Work out the finished part from the listing and answer in its coordinate system (mm). Face numbers are marked on the shaded views. A direction names the side the tool comes from. Round coordinates to 2 decimals unless told otherwise and drop trailing zeros. Write each loop counter-clockwise with the first axis right and the second up, starting at its lowest first coordinate (ties: lowest second). Pieces come first, ordered by that corner, then holes.
Autodesk Inventor part; units mm, degrees
ref_plane "YZ Plane" through (0, 0, 0) normal (1, 0, 0) x (0, 1, 0)
ref_plane "XZ Plane" through (0, 0, 0) normal (0, 1, 0) x (-1, 0, 0)
ref_plane "XY Plane" through (0, 0, 0) normal (0, 0, 1) x (1, 0, 0)
sketch "Sketch1" plane through (0, 0, 0) normal (0, 0, 1) x (1, 0, 0)
  circle A0 centre (0, 0) radius 17.399
  dimension "d0" = 34.798
extrude "Extrusion1" add sketch "Sketch1" against normal blind 30.734
sketch "Sketch2" plane through (0, 0, -30.734) normal (0, 0, -1) x (-1, 0, 0)
  circle A0 centre (0, 0) radius 18.415
  dimension "d3" = 36.83
extrude "Extrusion2" add sketch "Sketch2" along normal blind 20.066
sketch "Sketch3" plane through (0, 0, -50.8) normal (0, 0, -1) x (-1, 0, 0)
  line L0 (0, 0) -> (0, -7.112) construction
  circle A0 centre (0, -7.112) radius 5.969
  dimension "d6" = 7.112
  dimension "d7" = 11.938
extrude "Extrusion3" add sketch "Sketch3" along normal blind 6.096
sketch "Sketch4" plane through (0, -7.112, -56.896) normal (0, 0, -1) x (-1, 0, 0)
  circle A0 centre (0, 0) radius 3.048
  point P0 (0, 7.112)
  dimension "d10" = 6.096
extrude "Extrusion4" add sketch "Sketch4" along normal blind 16.002
properties part number "ShootingMech_Moter"
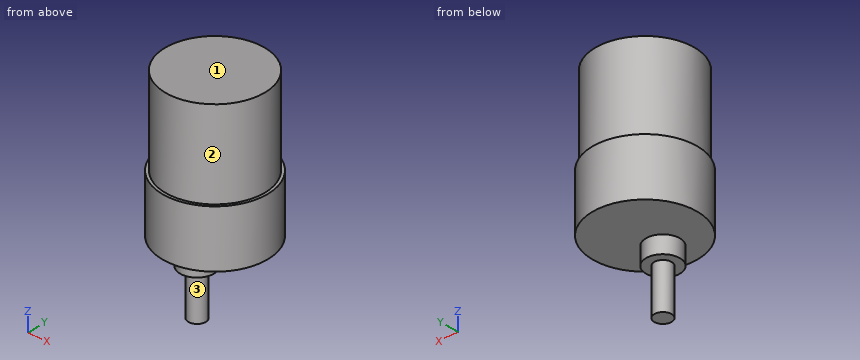
Q1. A tool of negligible diameter and unlimited length cuts with its end or side. For the marked faces 1, 2 and 3, from which of +Z, -Z, +X, -X, +Y, -Y can it reach the whole face along a straight path? Write none if from no direction.
Q2. Find section D-D (x = -8.5). Determine the outline of the cut face in (y, z).
Q3. Given pin 1 (12 mm diameter, centred on x = 7.5, y = 12.5, fed in from +Z); pin 2 (1.5 mm diameter, centred on x = 3.5, z = -36, fed in from -Y); pin 3 (1 mm diameter, centred on x = -9, z = -21.5, fed in from -Y); pin 4 (1 mm diameter, centred on y = 6.5, z = -16.5, fed in from +X), each flat-ended and moving along its own axis, determine where each tip first touches the part or whether it passes through.
Q4. Find section A-A (x = 0). Determine the outline of the cut face in (y, z) (3 decimals), plus the area to 3 significant figures.
Q5. Find section C-C (z = -12). Determine the outline of the cut face in (x, y), plus the area to 3 significant figures.
Q6. Find the intervals of material crossed by L1, parallel to Z at x = -13.5, y = 1; L2, parallel to Y at x = -6, z = -32; L3, parallel to X at y = 12.5, z = -41, in increasing order.
Q7. Find section B-B (y = 0). Determine the outline of the cut face in (x, z) (3 decimals).
Report:
1. face 1: +Z, +X, -X, +Y, -Y
1. face 2: +Z
1. face 3: -Z
2. outline: (-16.34, -50.8) - (16.34, -50.8) - (16.34, -30.73) - (15.18, -30.73) - (15.18, 0) - (-15.18, 0) - (-15.18, -30.73) - (-16.34, -30.73) - close
3. pin 1: stops at z = 0
3. pin 2: stops at y = -18.21
3. pin 3: stops at y = -15.18
3. pin 4: stops at x = 16.33
4. outline: (-18.415, -50.8) - (-13.081, -50.8) - (-13.081, -56.896) - (-10.16, -56.896) - (-10.16, -72.898) - (-4.064, -72.898) - (-4.064, -56.896) - (-1.143, -56.896) - (-1.143, -50.8) - (18.415, -50.8) - (18.415, -30.734) - (17.399, -30.734) - (17.399, 0) - (-17.399, 0) - (-17.399, -30.734) - (-18.415, -30.734) - close
4. area: 1,980 mm2
5. outline: circle Ø34.8 at (0, 0)
5. area: 951 mm2
6. L1: z = -50.8 to 0
6. L2: y = -17.41 to 17.41
6. L3: x = -13.52 to 13.52
7. outline: (-18.415, -50.8) - (18.415, -50.8) - (18.415, -30.734) - (17.399, -30.734) - (17.399, 0) - (-17.399, 0) - (-17.399, -30.734) - (-18.415, -30.734) - close
